from build123d import *

# Parameters (mm, degrees)
SKETCH_1_R          = 13
SKETCH_1_R_2        = 4.5
EXTRUDE_1_DEPTH     = 8
SKETCH_2_R          = 10.75
SKETCH_2_R_2        = 7.35
CUT_EXTRUDE_1_DEPTH = 1
CUT_EXTRUDE_START   = -1
SKETCH_3_R          = 10.75
SKETCH_3_R_2        = 7.35
CUT_EXTRUDE_2_DEPTH = 1


with BuildPart() as part:
    # Эскиз1 → Бобышка-Вытянуть1 (new body)
    with BuildSketch(Plane.XY):
        Circle(SKETCH_1_R)
        Circle(SKETCH_1_R_2, mode=Mode.SUBTRACT)
    extrude(amount=EXTRUDE_1_DEPTH)

    # Эскиз2 → Вырез-Вытянуть1 (cut)
    with BuildSketch(Plane.XY.offset(8)):
        Circle(SKETCH_2_R)
        Circle(SKETCH_2_R_2, mode=Mode.SUBTRACT)
    extrude(amount=-CUT_EXTRUDE_1_DEPTH, mode=Mode.SUBTRACT)

    # Эскиз3 → Вырез-Вытянуть2 (cut)
    with BuildSketch(Plane(origin=(0, 0, 0), x_dir=(-1, 0, 0), z_dir=(0, 0, -1)).offset(CUT_EXTRUDE_START)):
        with Locations(Location((0, 0, 0), (0, 0, 180))):
            Circle(SKETCH_3_R)
        with Locations(Location((0, 0, 0), (0, 0, 180))):
            Circle(SKETCH_3_R_2, mode=Mode.SUBTRACT)
    extrude(amount=CUT_EXTRUDE_2_DEPTH, mode=Mode.SUBTRACT)


solid = part.part
Work out the finished part from the listing and answer in its coordinate system (mm). A direction names the side the tool comes from. Coordinates: 2 decimals unless noted, no trailing zeros. Loops run counter-clockwise (first coordinate to the right, second up) from the corner with the lowest first, then second, coordinate; pieces in that order, holes last. Notation, with made-up numbers: M 61,70.5 L 98,70.5 A8 ccw 98,82.5 Z; hole C 48,39.5 d5. An arc over 180 degrees is marked long. Answer in a Markdown table with one row per item. Add a question column.
1. Find section C-C, the plane x = 2.5. Write down the section's boundary in (y, z), then the cut area to 3 significant figures.
2. Consider L1, parallel to Y at x = 0, z = 0.8; L2, parallel to Y at x = 0, z = 5.25; L3, parallel to Z at x = 3.75, y = -9.25. Determine where each line is inside the solid, lowest interval first.
3. The mould has two halves that part along X. Classify faces 4 (the cylindrical face through (-1.593, 7.175, 0.507)), 5 (the cylindrical face through (-10.316, -7.91, 3.944)), 6 (the flat face through (-5, 10, 8)): pulls with the +X half, pulls with the -X half, needs draft (parallel to the pull), parting line crosses it, or undercut.
4. Flat-ended cylindrical pins translate along their axes: P1, Ø3, axis at x = 6, z = 1, coming from the +Y side; P2, Ø1.5, axis at y = 5, z = 3.5, coming from the +X side; P3, Ø1.5, axis at y = -2.5, z = 5.5, coming from the +X side. Find the tip coordinate at first contact, or state that the pin passes through.
5. A tool of negligible diameter and unlimited length cuts with its end or side. For faces 1 (the flat face through (-5, 10, 0)), 2 (the cylindrical face through (-1.4, -10.66, 0.51)), 3 (the flat face through (-3, -7, 7)), from which of +Z, -Z, +X, -X, +Y, -Y can it reach the whole face along a straight path? Write none if from no direction.
6. Find section A-A, the plane y = 0. Write down the section's boundary in (x, z), then the cut area to 3 significant figures.
7. Find section B-B, the plane z = 7.5. Write down the section's boundary in (x, y), then the cut area to 3 significant figures.
8. Find section D-D, the plane z = 3.75. Write down the section's boundary in (x, y).
Reported:
| question | item | result |
|---|---|---|
| 1 | outline | M -12.76,0 L -10.46,0 L -10.46,1 L -6.91,1 L -6.91,0 L -3.74,0 L -3.74,8 L -6.91,8 L -6.91,7 L -10.46,7 L -10.46,8 L -12.76,8 Z; M 3.74,0 L 6.91,0 L 6.91,1 L 10.46,1 L 10.46,0 L 12.76,0 L 12.76,8 L 10.46,8 L 10.46,7 L 6.91,7 L 6.91,8 L 3.74,8 Z |
| 1 | area | 130 mm^2 |
| 2 | L1 | y = -13 to -10.75, -7.35 to -4.5, 4.5 to 7.35, 10.75 to 13 |
| 2 | L2 | y = -13 to -4.5, 4.5 to 13 |
| 2 | L3 | z = 1 to 7 |
| 3 | face 4 | undercut |
| 3 | face 5 | parting line crosses it |
| 3 | face 6 | needs draft |
| 4 | P1 | stops at y = 12.2 |
| 4 | P2 | stops at x = 12.29 |
| 4 | P3 | stops at x = 12.88 |
| 5 | face 1 | -Z, +X, -X, +Y, -Y |
| 5 | face 2 | -Z |
| 5 | face 3 | +Z |
| 6 | outline | M -13,0 L -10.75,0 L -10.75,1 L -7.35,1 L -7.35,0 L -4.5,0 L -4.5,8 L -7.35,8 L -7.35,7 L -10.75,7 L -10.75,8 L -13,8 Z; M 4.5,0 L 7.35,0 L 7.35,1 L 10.75,1 L 10.75,0 L 13,0 L 13,8 L 10.75,8 L 10.75,7 L 7.35,7 L 7.35,8 L 4.5,8 Z |
| 6 | area | 122 mm^2 |
| 7 | outline | C 0,0 d26; C 0,0 d14.7; hole C 0,0 d21.5; hole C 0,0 d9 |
| 7 | area | 274 mm^2 |
| 8 | outline | C 0,0 d26; hole C 0,0 d9 |
